from build123d import *

# Parameters (mm, degrees)
F0_W     = 25.4
F0_H     = 24.4
F0_R     = 2
F1_DEPTH = 1
F2_R     = 1.27
F3_W     = 25.4
F3_H     = 24.4
F3_R     = 1.5
F3_H_2   = 1
F4_DEPTH = 1
F5_R     = 1.27


with BuildPart() as f1:
    # F0 (on Front) → F1 (new body)
    with BuildSketch(Plane.XZ):
        Rectangle(F0_W, F0_H)
        Circle(F0_R, mode=Mode.SUBTRACT)
    extrude(amount=F1_DEPTH)

    # F2
    f2_edges = [f1.edges().sort_by_distance(p)[0] for p in [
        (12.7, -0.5, 12.2),
        (-12.7, -0.5, 12.2),
    ]]
    fillet(f2_edges, radius=F2_R)

    # F3 (on face) → F4 (join)
    with BuildSketch(Plane(origin=(0, 0, -12.2), x_dir=(1, 0, 0), z_dir=(0, 0, -1))):
        with Locations((0, -12.2)):
            Rectangle(F3_W, F3_H)
        with Locations((-6.35, -11.7)):
            Circle(F3_R, mode=Mode.SUBTRACT)
        with Locations((6.35, -11.7)):
            Circle(F3_R, mode=Mode.SUBTRACT)
        with Locations((0, 0.5)):
            Rectangle(F3_W, F3_H_2)
    extrude(amount=F4_DEPTH)

    # F5
    f5_edges = [f1.edges().sort_by_distance(p)[0] for p in [
        (0, -1, -13.2),
        (-12.7, 24.4, -12.7),
        (12.7, 24.4, -12.7),
    ]]
    fillet(f5_edges, radius=F5_R)


solid = f1.part
Verification items for the finished model (mm, model axes). A direction names the side the tool comes from. Round coordinates to 2 decimals unless told otherwise and drop trailing zeros. Loops run counter-clockwise (first coordinate to the right, second up) from the corner with the lowest first, then second, coordinate; pieces in that order, holes last. Notation, with made-up numbers: (37.5, 18.25) - (48.5, 18.25) arc R21 ccw to (48.5, 44.25) - close; hole circle Ø1 at (20.5, -5.5). An arc over 180 degrees is marked (long way). Write item = value, one per line.
Q1. Sectioned sample at A-A on z = 0. Record the boundary of the cut face in (x, y).
Here are the results:
outline = (-12.7, -1) - (-2, -1) - (-2, 0) - (-12.7, 0) - close; (2, -1) - (12.7, -1) - (12.7, 0) - (2, 0) - close
Q2. Sectioned sample at D-D on x = -9. Record the boundary of the cut face in (y, z).
Here are the results:
outline = (-1, -11.93) arc R1.27 ccw to (0.27, -13.2) - (24.4, -13.2) - (24.4, -12.2) - (0, -12.2) - (0, 12.2) - (-1, 12.2) - close
Q3. Mould release check, pull along Y, two halves, no side actions. Record for faces 3 (the flat face through (0, 0, 3)), 4 (the cylindrical face through (12.318, -0.507, 11.838)), 5 (the cylindrical face through (6.025, 13.164, -12.693)): +Y half, -Y half, draft (parallel to the pull), parting line (faces both ways), or undercut.
Here are the results:
face_3 = +Y half
face_4 = draft
face_5 = undercut
Q4. Sectioned sample at B-B on y = 11.7. Record the boundary of the cut face in (x, z).
Here are the results:
outline = (-12.7, -13.2) - (-7.85, -13.2) - (-7.85, -12.2) - (-12.7, -12.2) - close; (-4.85, -13.2) - (4.85, -13.2) - (4.85, -12.2) - (-4.85, -12.2) - close; (7.85, -13.2) - (12.7, -13.2) - (12.7, -12.2) - (7.85, -12.2) - close
Q5. Sectioned sample at C-C on x = 0. Record the boundary of the cut face in (y, z), plus the area to 3 significant figures.
Here are the results:
outline = (-1, -11.93) arc R1.27 ccw to (0.27, -13.2) - (24.4, -13.2) - (24.4, -12.2) - (0, -12.2) - (0, -2) - (-1, -2) - close; (-1, 2) - (0, 2) - (0, 12.2) - (-1, 12.2) - close
area = 45.5 mm^2
Q6. Material ranges on L1, parallel to X at y = 11.7, z = -12.55; L2, parallel to Z at x = -3, y = 3.5; L3, parallel to Z at x = 0, y = -0.7, recorded low to high.
Here are the results:
L1 = -12.7 to -7.85, -4.85 to 4.85, 7.85 to 12.7
L2 = -13.2 to -12.2
L3 = -12.75 to -2, 2 to 12.2
Q7. Tool access check on faces 1 (the flat face through (0, 12, -12.2)), 2 (the flat face through (-0.2, -0.5, 12.2)). Record the directions out of +Z, -Z, +X, -X, +Y, -Y that give a thin tool (end or side, any length) a straight path to the whole face; none if there is none.
Here are the results:
face_1 = +Z, +X, -X, +Y
face_2 = +Z, +X, -X, +Y, -Y
Q8. Depth check by flat-ended pin: pin 1 (1.5 mm diameter, centred on x = 1, z = 4, fed in from +Y); pin 2 (12 mm diameter, centred on x = -8.5, y = 12, fed in from +Z); pin 3 (4 mm diameter, centred on x = -6.35, y = 11.7, fed in from -Z). Enter the tip coordinate at first touch or a pass-through.
Here are the results:
pin_1 = 0
pin_2 = -12.2
pin_3 = -13.2
